from build123d import *

# Parameters (mm, degrees)
F0_W     = 390
F0_H     = 300
F0_W_2   = 129.2868405581
F0_H_2   = 32.5715690851
F1_DEPTH = 50
F2_W     = 129.2868405581
F2_H     = 22.3345696926
F3_DEPTH = 25
F4_R     = 10


# Not quite as in the source:
# - a pattern or mirror of a feature is missing from the dataset's text; its kind, count and spacing are read off the source's solid


with BuildPart() as f1:
    # F0 (on Front) → F1 (new body, symmetric)
    with BuildSketch(Plane.XZ):
        Rectangle(F0_W, F0_H)
        with Locations((0, 111.3796457648)):
            Rectangle(F0_W_2, F0_H_2, mode=Mode.SUBTRACT)
    extrude(amount=F1_DEPTH, both=True)

    # F2 (on face) → F3 (cut)
    with BuildSketch(Plane.XZ.offset(50)):
        with Locations((0, 138.8327151537)):
            Rectangle(F2_W, F2_H)
    f3 = extrude(amount=-F3_DEPTH, mode=Mode.SUBTRACT)

    # F3_copies: F3 across plane
    add(f3.mirror(Plane.ZX), mode=Mode.SUBTRACT)

    # F4
    f4_edges = [f1.edges().sort_by_distance(p)[0] for p in [
        (0, -50, -150),
        (195, -50, 0),
        (129.82171, -50, 150),
        (64.64342, -50, 122.546931),
        (0, -50, 95.093861),
        (-64.64342, -50, 122.546931),
        (-129.82171, -50, 150),
        (-195, -50, 0),
        (-195, 0, 150),
        (-195, 50, 0),
        (-195, 0, -150),
        (195, 0, 150),
        (64.64342, -37.5, 150),
        (0, -25, 150),
        (-64.64342, -37.5, 150),
        (-129.82171, 50, 150),
        (-64.64342, 37.5, 150),
        (0, 25, 150),
        (64.64342, 37.5, 150),
        (129.82171, 50, 150),
        (0, 50, -150),
        (195, 50, 0),
        (64.64342, 50, 122.546931),
        (0, 50, 95.093861),
        (-64.64342, 50, 122.546931),
        (195, 0, -150),
    ]]
    fillet(f4_edges, radius=F4_R)


solid = f1.part
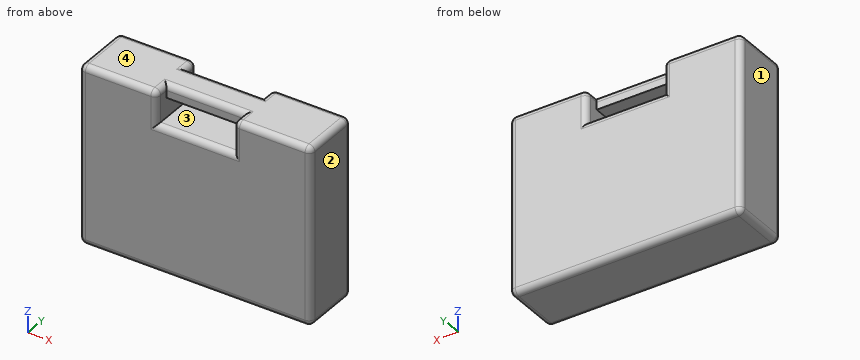
Work out the finished part from the listing and answer in its coordinate system (mm). Face numbers are marked on the shaded views. Coordinates: 2 decimals unless noted, no trailing zeros. Loops run counter-clockwise (first coordinate to the right, second up) from the corner with the lowest first, then second, coordinate; pieces in that order, holes last. Notation, with made-up numbers: (-23, -8) -> (6, -8) arc R31 cw to (6, 17) -> close; hole circle Ø8 at (41, 40.5). An arc over 180 degrees is marked (long way). Write each question's results on one line, items separated by ' | '. Start each with the question number.
1) Consider line 1 along X through (y, z) = (-27, 95.5); line 2 along Z through (x, y) = (-23.5, -10.5); line 3 along X through (y, z) = (41, 20). Determine where each line is inside the solid, lowest interval first.
2) Find section A-A on z = 115. Determine the outline of the cut face in (x, y).
3) Flat-ended cylindrical pins translate along their axes: P1, Ø6, axis at x = -26, z = 134.5, coming from the -Y side; P2, Ø6, axis at x = -4, z = 135, coming from the +Y side. Find the tip coordinate at first contact, or state that the pin passes through.
4) Find section B-B on y = -5. Determine the outline of the cut face in (x, z).
5) The mould has two halves that part along X. Classify the marked faces 1, 2, 3 and 4: pulls with the +X half, pulls with the -X half, needs draft (parallel to the pull), parting line crosses it, or undercut.
6) Find section C-C on x = 54. Determine the outline of the cut face in (y, z), then the cut area to 3 significant figures.
Response values:
1) line 1: x = -195 to -64.64, 64.64 to 195 | line 2: z = -150 to 95.09, 127.67 to 150 | line 3: x = -194.95 to 194.95
2) outline: (-195, -40) arc R10 ccw to (-185, -50) -> (-74.64, -50) arc R10 ccw to (-64.64, -40) -> (-64.64, 40) arc R10 ccw to (-74.64, 50) -> (-185, 50) arc R10 ccw to (-195, 40) -> close; (64.64, -40) arc R10 ccw to (74.64, -50) -> (185, -50) arc R10 ccw to (195, -40) -> (195, 40) arc R10 ccw to (185, 50) -> (74.64, 50) arc R10 ccw to (64.64, 40) -> close
3) P1: stops at y = -25 | P2: stops at y = 25
4) outline: (-195, -140) arc R10 ccw to (-185, -150) -> (185, -150) arc R10 ccw to (195, -140) -> (195, 140) arc R10 ccw to (185, 150) -> (-185, 150) arc R10 ccw to (-195, 140) -> close; hole (-64.64, 95.09) -> (64.64, 95.09) -> (64.64, 127.67) -> (-64.64, 127.67) -> close
5) face 1: pulls with the -X half | face 2: pulls with the +X half | face 3: undercut | face 4: needs draft
6) outline: (-50, -140) arc R10 ccw to (-40, -150) -> (40, -150) arc R10 ccw to (50, -140) -> (50, 85.09) arc R10 ccw to (40, 95.09) -> (-40, 95.09) arc R10 ccw to (-50, 85.09) -> close; (-25, 127.67) -> (25, 127.67) -> (25, 140) arc R10 ccw to (15, 150) -> (-15, 150) arc R10 ccw to (-25, 140) -> close | area: 25,500 mm^2
